```python
from build123d import *

# Parameters (mm, degrees)
BOSS_EXTRUDE2_DEPTH = 20
SKETCH2_R           = 2.55
CUT_EXTRUDE1_DEPTH  = 20
FILLET1_R           = 1


with BuildPart() as part:
    # Sketch1 → Boss-Extrude2 (new body)
    with BuildSketch(Plane(origin=(0, 0, 0), x_dir=(1, 0, 0), z_dir=(0, 1, 0))):
        with BuildLine():
            Line((7.5, 0), (19.5, 0))
            ThreePointArc((19.5, 0), (13.788582233, 13.788582233), (0, 19.5))
            Line((0, 19.5), (0, 7.5))
            ThreePointArc((0, 7.5), (-5.303300859, -5.303300859), (7.5, 0))
        make_face()
    extrude(amount=BOSS_EXTRUDE2_DEPTH)

    # Sketch2 → Cut-Extrude1 (cut)
    with BuildSketch(Plane(origin=(0, 20, 0), x_dir=(1, 0, 0), z_dir=(0, 1, 0))):
        with Locations(Location((0, 0, 0), (0, 0, 270))):
            Circle(SKETCH2_R)
    extrude(amount=-CUT_EXTRUDE1_DEPTH, mode=Mode.SUBTRACT)

    # Fillet1
    fillet1_edges = [part.edges().sort_by_distance(p)[0] for p in [
        (0, 10, -7.5),
        (0, 10, -19.5),
        (19.5, 10, 0),
        (7.5, 10, 0),
    ]]
    fillet(fillet1_edges, radius=FILLET1_R)


solid = part.part
```
Can you work these out from the model? Positions are in its coordinate system, mm. A direction names the side the tool comes from. Give positions to 0.01 mm unless a question says otherwise; leave off trailing zeros. Write each loop counter-clockwise with the first axis right and the second up, starting at its lowest first coordinate (ties: lowest second). Pieces come first, ordered by that corner, then holes. Notation, with made-up numbers: (4.25, 14.5) - (44.25, 14.5) arc R20 ccw to (44.25, 26.5) - close; hole circle Ø6 at (-35.75, 38.25). An arc over 180 degrees is marked (long way). Write item = value, one per line. Start each with the question number.
1. Please list where these lines run through material, in increasing order: line 1 (X direction, y = 8, z = -12.5); line 2 (Z direction, x = -5.25, y = 17); line 3 (X direction, y = 6.25, z = -8).
2. On a 3-axis mill with a long thin cutter (end or side, diameter ignored), from which of +Z, -Z, +X, -X, +Y, -Y can I reach the whole of each face in a straight line? I mean faces 1 (the face through (6, 0, -6)), 2 (the face through (13, 10, 0)). Say none if no direction works.
3. Imagine slicing it at C-C (z = -17.5). Please give me the cut outline in (x, y), and give its area (3 significant figures).
4. Thinking about a two-plate mould opening in X: for faces 3 (the face through (7.78, 10.14, 0.25)), 4 (the face through (0, 10, -14)), 5 (the face through (0.77, 10.14, 2.43)), which applies, released by +X, released by -X, zero draft, split by the parting line, or undercut?
5. For pin 1 (5 mm diameter, centred on y = 15.5, z = -6.5, fed in from -X); pin 2 (6 mm diameter, centred on x = 5.5, y = 7.5, fed in from +Z); pin 3 (4 mm diameter, centred on y = 14.5, z = -4.5, fed in from -X), each with a flat end and sliding along its axis, tell me the tip position at first contact or that it passes through.
6. Imagine slicing it at B-B (x = 14). Please give me the cut outline in (y, z), and give its area (3 significant figures).
7. Imagine slicing it at A-A (y = 3.75). Please give me the cut outline in (x, z).
Worked answers:
q1.line_1 = 0 to 14.97
q1.line_2 = -5.36 to 5.36
q1.line_3 = -0.1 to 17.78
q2.face_1 = +Z, -Z, +X, -X, -Y
q2.face_2 = +Z, +X, +Y, -Y
q3.outline = (0, 0) - (8.6, 0) - (8.6, 20) - (0, 20) - close
q3.area = 172 mm2
q4.face_3 = released by +X
q4.face_4 = released by -X
q4.face_5 = undercut
q5.pin_1 = -6.34
q5.pin_2 = 7.07
q5.pin_3 = -7.07
q6.outline = (0, -13.57) - (20, -13.57) - (20, 0) - (0, 0) - close
q6.area = 271 mm2
q7.outline = (-0.88, -7.45) arc R1 cw to (0, -8.44) - (0, -18.47) arc R1 ccw to (1.05, -19.47) arc R19.5 ccw to (19.47, -1.05) arc R1 ccw to (18.47, 0) - (8.44, 0) arc R1 cw to (7.45, 0.88) arc R7.5 ccw (long way) to start; hole circle Ø5.1 at (0, 0)
